Verification items for the finished model (mm, model axes). A direction names the side the tool comes from. Round coordinates to 2 decimals unless told otherwise and drop trailing zeros. Order: outer loops, then holes, each group sorted by start corner. A loop starts at its lowest first (then second) coordinate and runs counter-clockwise, first axis right, second up. Notation, with made-up numbers: M 60.25,7.5 L 89.25,7.5 A10 ccw 89.25,25.5 Z; hole C -22,-1 d2. An arc over 180 degrees is marked long. Write item = value, one per line. Start each with the question number.
from build123d import *

# Parameters (mm, degrees)
SKETCH1_W           = 33
SKETCH1_H           = 33
SKETCH1_W_2         = 23
SKETCH1_H_2         = 13
BOSS_EXTRUDE1_DEPTH = 2
CHAMFER1_SIZE       = 0.5
CHAMFER1_SIZE2      = 0.866025404
SKETCH2_W           = 33
SKETCH2_H           = 33
SKETCH2_W_2         = 27
SKETCH2_H_2         = 28.15
BOSS_EXTRUDE2_DEPTH = 3
CUT_EXTRUDE2_DEPTH  = 3
SKETCH4_R           = 1.9
SKETCH4_R_2         = 1.1
BOSS_EXTRUDE3_DEPTH = 1.5
CUT_EXTRUDE3_START  = -10
SKETCH5_R           = 1.35
CUT_EXTRUDE3_DEPTH  = 10
SKETCH6_W           = 15
SKETCH6_H           = 1.5
CUT_EXTRUDE4_DEPTH  = 3


with BuildPart() as part:
    # Sketch1 → Boss-Extrude1 (new body)
    with BuildSketch(Plane.XY):
        with Locations((-0.6, 1.925)):
            Rectangle(SKETCH1_W, SKETCH1_H)
        with Locations((-0.6, -0.075)):
            Rectangle(SKETCH1_W_2, SKETCH1_H_2, mode=Mode.SUBTRACT)
    extrude(amount=BOSS_EXTRUDE1_DEPTH)

    # Chamfer1
    chamfer1_edges = [part.edges().sort_by_distance(p)[0] for p in [
        (-12.1, -0.075, 2),
        (-0.6, -6.575, 2),
        (10.9, -0.075, 2),
        (-0.6, 6.425, 2),
    ]]
    chamfer1_side = [part.faces().sort_by_distance(p)[0] for p in [
        (-0.6, -14.108309524, 2),
    ]]
    chamfer(chamfer1_edges, length=CHAMFER1_SIZE, length2=CHAMFER1_SIZE2, reference=chamfer1_side[0])

    # Sketch2 → Boss-Extrude2 (add)
    with BuildSketch(Plane(origin=(0, 0, 0), x_dir=(-1, 0, 0), z_dir=(0, 0, -1))):
        with Locations((0.6, 1.925)):
            Rectangle(SKETCH2_W, SKETCH2_H)
        with Locations((0.6, 2)):
            Rectangle(SKETCH2_W_2, SKETCH2_H_2, mode=Mode.SUBTRACT)
    extrude(amount=BOSS_EXTRUDE2_DEPTH)

    # Sketch3 → Cut-Extrude2 (cut)
    with BuildSketch(Plane(origin=(0, 0, 0), x_dir=(-1, 0, 0), z_dir=(0, 0, -1))):
        with BuildLine():
            Line((-10.95, 12.725), (-10.95, 14.075))
            Line((-10.95, 14.075), (-9.6, 14.075))
            ThreePointArc((-9.6, 14.075), (-11.904594155, 15.029594155), (-10.95, 12.725))
        make_face()
        with BuildLine():
            Line((-9.6, 14.075), (-10.95, 14.075))
            Line((-10.95, 14.075), (-10.95, 12.725))
            ThreePointArc((-10.95, 12.725), (-9.995405845, 13.120405845), (-9.6, 14.075))
        make_face()
        with BuildLine():
            ThreePointArc((13.5, 14.075), (12.15, 15.425), (10.8, 14.075))
            Line((10.8, 14.075), (12.15, 14.075))
            Line((12.15, 14.075), (12.15, 12.725))
            ThreePointArc((12.15, 12.725), (13.104594155, 13.120405845), (13.5, 14.075))
        make_face()
        with BuildLine():
            Line((12.15, 14.075), (10.8, 14.075))
            ThreePointArc((10.8, 14.075), (11.195405845, 13.120405845), (12.15, 12.725))
            Line((12.15, 12.725), (12.15, 14.075))
        make_face()
        with BuildLine():
            ThreePointArc((13.5, -9.425), (13.104594155, -8.470405845), (12.15, -8.075))
            Line((12.15, -8.075), (12.15, -9.425))
            Line((12.15, -9.425), (10.8, -9.425))
            ThreePointArc((10.8, -9.425), (12.15, -10.775), (13.5, -9.425))
        make_face()
        with BuildLine():
            Line((12.15, -9.425), (12.15, -8.075))
            ThreePointArc((12.15, -8.075), (11.195405845, -8.470405845), (10.8, -9.425))
            Line((10.8, -9.425), (12.15, -9.425))
        make_face()
        with BuildLine():
            ThreePointArc((-9.6, -9.425), (-9.995405845, -8.470405845), (-10.95, -8.075))
            Line((-10.95, -8.075), (-10.95, -9.425))
            Line((-10.95, -9.425), (-9.6, -9.425))
        make_face()
        with BuildLine():
            Line((-10.95, -9.425), (-10.95, -8.075))
            ThreePointArc((-10.95, -8.075), (-11.904594155, -10.379594155), (-9.6, -9.425))
            Line((-9.6, -9.425), (-10.95, -9.425))
        make_face()
    extrude(amount=-CUT_EXTRUDE2_DEPTH, mode=Mode.SUBTRACT)

    # Sketch4 → Boss-Extrude3 (add)
    # profile 1 of 4: a face of its own
    with BuildSketch(Plane(origin=(0, 0, 0), x_dir=(-1, 0, 0), z_dir=(0, 0, -1))):
        with Locations((-10.95, 14.075)):
            Circle(SKETCH4_R)
        with Locations((-10.95, 14.075)):
            Circle(SKETCH4_R_2, mode=Mode.SUBTRACT)
    # profile 2 of 4: a face of its own
    with BuildSketch(Plane(origin=(0, 0, 0), x_dir=(-1, 0, 0), z_dir=(0, 0, -1))):
        with Locations((12.15, 14.075)):
            Circle(SKETCH4_R)
        with Locations((12.15, 14.075)):
            Circle(SKETCH4_R_2, mode=Mode.SUBTRACT)
    # profile 3 of 4: a face of its own
    with BuildSketch(Plane(origin=(0, 0, 0), x_dir=(-1, 0, 0), z_dir=(0, 0, -1))):
        with Locations((-10.95, -9.425)):
            Circle(SKETCH4_R)
        with Locations((-10.95, -9.425)):
            Circle(SKETCH4_R_2, mode=Mode.SUBTRACT)
    # profile 4 of 4: a face of its own
    with BuildSketch(Plane(origin=(0, 0, 0), x_dir=(-1, 0, 0), z_dir=(0, 0, -1))):
        with Locations((12.15, -9.425)):
            Circle(SKETCH4_R)
        with Locations((12.15, -9.425)):
            Circle(SKETCH4_R_2, mode=Mode.SUBTRACT)
    extrude(amount=BOSS_EXTRUDE3_DEPTH)

    # Sketch5 → Cut-Extrude3 (cut)
    with BuildSketch(Plane.XY.offset(2).offset(CUT_EXTRUDE3_START)):
        with Locations(Location((-12.15, 14.075, 0), (0, 0, 180))):
            Circle(SKETCH5_R)
        with Locations(Location((10.95, 14.075, 0), (0, 0, 180))):
            Circle(SKETCH5_R)
        with Locations(Location((-12.15, -9.425, 0), (0, 0, 180))):
            Circle(SKETCH5_R)
        with Locations(Location((10.95, -9.425, 0), (0, 0, 180))):
            Circle(SKETCH5_R)
    extrude(amount=CUT_EXTRUDE3_DEPTH, mode=Mode.SUBTRACT)

    # Sketch6 → Cut-Extrude4 (cut)
    with BuildSketch(Plane(origin=(0, 0, -3), x_dir=(-1, 0, 0), z_dir=(0, 0, -1))):
        with Locations((0.6, -12.825)):
            Rectangle(SKETCH6_W, SKETCH6_H)
    extrude(amount=-CUT_EXTRUDE4_DEPTH, mode=Mode.SUBTRACT)


solid = part.part
1) Scan lines: probe 1 along Y at (x, z) = (10.95, 1) (3 decimals); probe 2 along Y at (x, z) = (5.5, -2.15) (3 decimals); probe 3 along X at (y, z) = (11.5, -1.4). Record each from-to range of solid material in increasing order.
2) Gauge pin test, flat ends, axial feed: P1, Ø1.6, axis at x = 10.95, y = -9.425, coming from the -Z side; P2, Ø3, axis at x = -12.5, y = -9, coming from the -Z side. Record the tip position at first contact, or that the pin passes through.
3) Access from +Z, -Z, +X, -X, +Y, -Y to the whole of each face (thin tool, end or side, straight path). Record for faces 4 (the flat face through (-12.346, -0.173, 1.561)), 5 (the flat face through (-8.1, -13, -2)), 6 (the flat face through (10.9, -0.2, 0.6)), 7 (the flat face through (0, 18.425, 0)), 8 (the flat face through (-1, 9, 2)).
4) Cross-section at B-B, the plane x = 3. Enter the section's corners in (y, z) (3 decimals).
5) Cross-section at A-A, the plane z = -0.4. Give the number of separate pieces and of enclosed holes in the cut face, then the cut area to 3 significant figures.
6) Release check for a two-part mould opening along X. For faces 1 (the flat face through (-17.1, 2, 0)), 2 (the flat face through (0, -14.575, 0)), 3 (the flat face through (10, -12.075, -1)) record: pulls with the +X half, pulls with the -X half, needs draft (parallel to the pull), parting line crosses it, or undercut.
7) Cross-section at D-D, the plane y = 3. Enter the section's corners in (x, z), then the cut area to 3 significant figures.
8) Cross-section at C-C, the plane y = -9. Enter the section's corners in (x, z), then the cut area to 3 significant figures.
Geometry results:
q1.probe_1 = -14.575 to -10.775, -8.075 to 12.725, 15.425 to 18.425
q1.probe_2 = -14.575 to -13.575, 16.075 to 18.425
q1.probe_3 = -17.1 to -14.1, 12.9 to 15.9
q2.P1 = through
q2.P2 = -1.5
q3.face_4 = +Z
q3.face_5 = -Z
q3.face_6 = +Z, -Z
q3.face_7 = +Z, -Z, +X, -X, +Y
q3.face_8 = +Z, +X, -X, +Y, -Y
q4.outline = M -14.575,-3 L -13.575,-3 L -13.575,0 L -6.575,0 L -6.575,1.134 L -7.075,2 L -14.575,2 Z; M 6.425,0 L 16.075,0 L 16.075,-3 L 18.425,-3 L 18.425,2 L 6.925,2 L 6.425,1.134 Z
q5.separate_pieces = 5
q5.enclosed_holes = 5
q5.area = 329 mm^2
q6.face_1 = pulls with the -X half
q6.face_2 = needs draft
q6.face_3 = undercut
q7.outline = M -17.1,-3 L -14.1,-3 L -14.1,0 L -12.1,0 L -12.1,1.13 L -12.6,2 L -17.1,2 Z; M 10.9,0 L 12.9,0 L 12.9,-3 L 15.9,-3 L 15.9,2 L 11.4,2 L 10.9,1.13 Z
q7.area = 37.6 mm^2
q8.outline = M -17.1,-3 L -14.1,-3 L -14.1,0 L -14,0 L -14,-1.5 L -13.43,-1.5 L -13.43,2 L -17.1,2 Z; M -10.87,-1.5 L -10.3,-1.5 L -10.3,0 L 9.1,0 L 9.1,-1.5 L 9.67,-1.5 L 9.67,2 L -10.87,2 Z; M 12.23,-1.5 L 12.8,-1.5 L 12.8,0 L 12.9,0 L 12.9,-3 L 15.9,-3 L 15.9,2 L 12.23,2 Z
q8.area = 77.2 mm^2
